from build123d import *

# Parameters (mm, degrees)
SKETCH1_W           = 20
SKETCH1_H           = 20
BOSS_EXTRUDE1_DEPTH = 20
CUT_EXTRUDE1_DEPTH  = 20
CUT_EXTRUDE2_DEPTH  = 20
CUT_EXTRUDE3_DEPTH  = 20
CUT_EXTRUDE4_DEPTH  = 20


with BuildPart() as part:
    # Sketch1 → Boss-Extrude1 (new body)
    with BuildSketch(Plane.XY):
        with Locations((10, 10)):
            Rectangle(SKETCH1_W, SKETCH1_H)
    extrude(amount=BOSS_EXTRUDE1_DEPTH)

    # Sketch2 → Cut-Extrude1 (cut)
    with BuildSketch(Plane(origin=(0, 20, 0), x_dir=(1, 0, 0), z_dir=(0, 1, 0))):
        Polygon((20, 0), (10, 0), (20, -10), align=None)
    extrude(amount=-CUT_EXTRUDE1_DEPTH, mode=Mode.SUBTRACT)

    # Sketch3 → Cut-Extrude2 (cut)
    with BuildSketch(Plane(origin=(0, 20, 0), x_dir=(1, 0, 0), z_dir=(0, 1, 0))):
        Polygon((20, -20), (10, -20), (20, -10), align=None)
    extrude(amount=-CUT_EXTRUDE2_DEPTH, mode=Mode.SUBTRACT)

    # Sketch4 → Cut-Extrude3 (cut)
    with BuildSketch(Plane(origin=(0, 20, 0), x_dir=(1, 0, 0), z_dir=(0, 1, 0))):
        Polygon((10, -20), (0, -10), (0, -20), align=None)
    extrude(amount=-CUT_EXTRUDE3_DEPTH, mode=Mode.SUBTRACT)

    # Sketch5 → Cut-Extrude4 (cut)
    with BuildSketch(Plane(origin=(0, 20, 0), x_dir=(1, 0, 0), z_dir=(0, 1, 0))):
        Polygon((10, 0), (0, -5), (0, 0), align=None)
    extrude(amount=-CUT_EXTRUDE4_DEPTH, mode=Mode.SUBTRACT)


solid = part.part
Source: CAD feature listing. Evaluate the final solid. Frame: model axes, mm. Coordinates: 2 decimals unless noted, no trailing zeros. Loops run counter-clockwise (first coordinate to the right, second up) from the corner with the lowest first, then second, coordinate; pieces in that order, holes last. Notation, with made-up numbers: (52.5, 76.25) - (97.5, 76.25) arc R19 ccw to (97.5, 103.25) - close; hole circle Ø9 at (-31.75, 8.5). An arc over 180 degrees is marked (long way). One line per item, written item: value. Start each with the question number.
1. Contact query for flat-ended pins moving along their axis: P1, Ø1.5, axis at y = 4, z = 13, coming from the -X side; P2, Ø2, axis at x = 14.5, y = 9.5, coming from the +Z side. Output: stop coordinate, or through.
2. Section C-C (y = 2). Return the cut outline in (x, z), and give its area (3 significant figures).
3. Ray query, L1, parallel to Z at x = 17, y = 18; L2, parallel to X at y = 16, z = 6.5; L3, parallel to Z at x = 18, y = 10.5. Return the intervals inside material, ascending.
4. Section B-B (z = 9). Return the cut outline in (x, y).
5. Section A-A (x = 6). Return the cut outline in (y, z), and give its area (3 significant figures).
Verdict:
1. P1: stops at x = 2.25
1. P2: stops at z = 16.5
2. outline: (0, 5) - (10, 0) - (20, 10) - (10, 20) - (0, 10) - close
2. area: 225 mm2
3. L1: z = 7 to 13
3. L2: x = 0 to 16.5
3. L3: z = 8 to 12
4. outline: (0, 0) - (19, 0) - (19, 20) - (0, 20) - close
5. outline: (0, 2) - (20, 2) - (20, 16) - (0, 16) - close
5. area: 280 mm2
